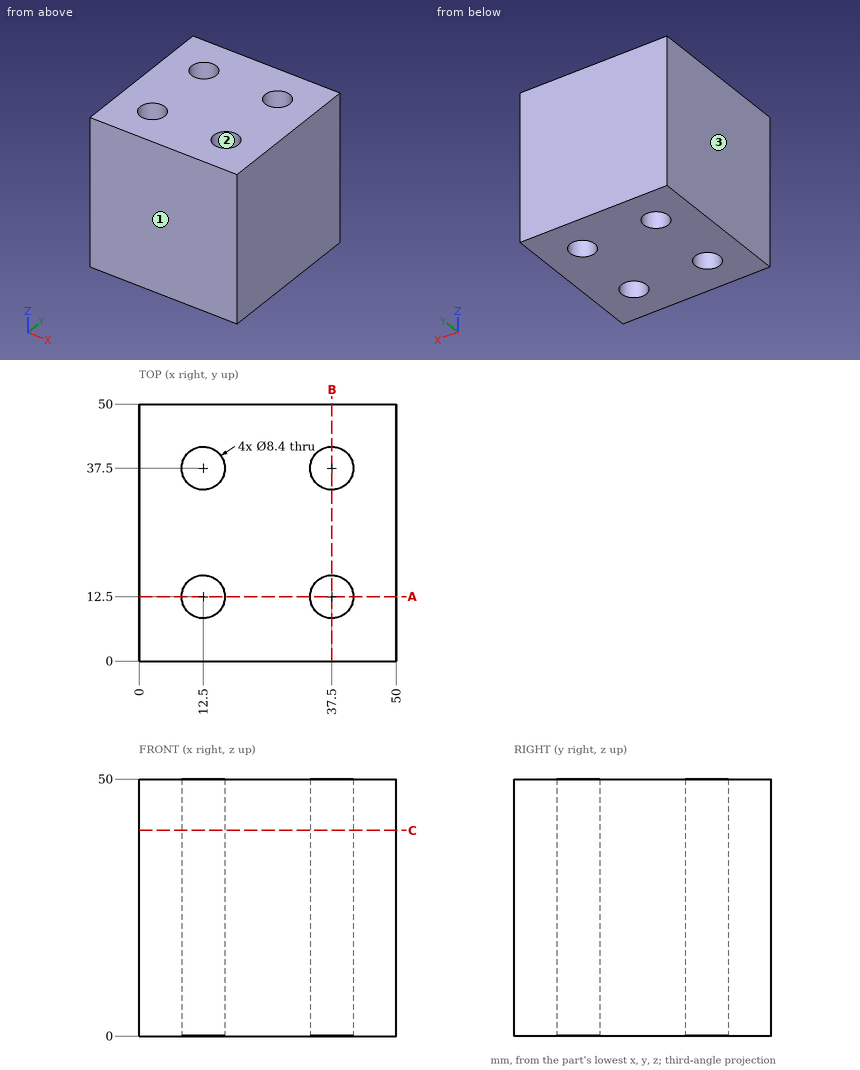
Check sheet for the drawn part. Datum: minimum x, y, z corner. Units: mm. Give positions to 0.01 mm unless a question says otherwise; leave off trailing zeros. Order: outer loops, then holes, each group sorted by start corner. A loop starts at its lowest first (then second) coordinate and runs counter-clockwise, first axis right, second up. Notation, with made-up numbers: (-31, 28.25) -> (-15, 28.25) arc R13 cw to (-15, 36.25) -> close; hole circle Ø1 at (-1.75, 15). An arc over 180 degrees is marked (long way). Return JSON: item names as keys, results as strings.
1. Mould release check, pull along Y, two halves, no side actions. Record for the marked faces 1, 2 and 3: +Y half, -Y half, draft (parallel to the pull), parting line (faces both ways), or undercut.
From the geometry:
{"face 1": "-Y half", "face 2": "undercut", "face 3": "draft"}
2. Cross-section at C-C, the plane z = 40. Record the cut outline in (x, y), plus the area to 3 significant figures.
From the geometry:
{"outline": "(0, 0) -> (50, 0) -> (50, 50) -> (0, 50) -> close; hole circle Ø8.4 at (12.5, 12.5); hole circle Ø8.4 at (12.5, 37.5); hole circle Ø8.4 at (37.5, 12.5); hole circle Ø8.4 at (37.5, 37.5)", "area": "2,280 mm^2"}
3. Material ranges on probe 1 along Y at (x, z) = (12.5, 27.5); probe 2 along Y at (x, z) = (10, 44); probe 3 along X at (y, z) = (14.5, 32.5), recorded low to high. Write a range as [from, to].
From the geometry:
{"probe 1": "[0, 8.3], [16.7, 33.3], [41.7, 50]", "probe 2": "[0, 9.13], [15.87, 34.13], [40.87, 50]", "probe 3": "[0, 8.81], [16.19, 33.81], [41.19, 50]"}
4. Cross-section at A-A, the plane y = 12.5. Record the cut outline in (x, z).
From the geometry:
{"outline": "(0, 0) -> (8.3, 0) -> (8.3, 50) -> (0, 50) -> close; (16.7, 0) -> (33.3, 0) -> (33.3, 50) -> (16.7, 50) -> close; (41.7, 0) -> (50, 0) -> (50, 50) -> (41.7, 50) -> close"}
